Design review of the part built by this model. Coordinates are the model's own, in mm. Coordinates: 2 decimals unless noted, no trailing zeros. Loops run counter-clockwise (first coordinate to the right, second up) from the corner with the lowest first, then second, coordinate; pieces in that order, holes last. Notation, with made-up numbers: M -6,6 L 1,6 A20 ccw 1,32 Z; hole C 43,-1 d8. An arc over 180 degrees is marked long. Answer as a JSON object with one key per item and string values. Group by question number.
1. Consider section C-C (y = 5.5). State the section outline as (x, z) points (3 decimals).
2. Insertion check: pin 1 (0.8 mm diameter, centred on x = 93.5, z = 2.5, fed in from -Y); pin 2 (1 mm diameter, centred on y = 23.5, z = 1, fed in from +X); pin 3 (1 mm diameter, centred on x = 139.5, z = 1.5, fed in from +Y); pin 4 (3.5 mm diameter, centred on x = 104.67, y = 62.3, fed in from +Z) (3 decimals). Each pin has a flat end and moves straight along its axis. Give the tip position at first contact, or say it passes through.
3. To check wall thickness, follow probe 1 along Y at (x, z) = (149, 0.4); probe 2 along Y at (x, z) = (93.5, 1.4); probe 3 along X at (y, z) = (22, 2.05). State the ranges of each line that lie inside material, in increasing order.
4. Consider section B-B (x = 129). State the section outline as (y, z) points (3 decimals), then the cut area to 3 significant figures.
from build123d import *

# Parameters (mm, degrees)
SKETCH1_R           = 1.5875
BOSS_EXTRUDE1_DEPTH = 3.175


with BuildPart() as part:
    # Sketch1 → Boss-Extrude1 (new body)
    with BuildSketch(Plane.XY):
        with BuildLine():
            Line((145.943650407, -28.027444193), (145.943650407, -24.852444193))
            Line((145.943650407, -24.852444193), (152.293650407, -24.852444193))
            Line((152.293650407, -24.852444193), (155.468650407, -24.852444193))
            Line((155.468650407, -24.852444193), (155.468650407, -28.027444193))
            Line((155.468650407, -28.027444193), (155.468650407, -40.727444193))
            Line((155.468650407, -40.727444193), (155.468650407, -43.902444193))
            Line((155.468650407, -43.902444193), (145.943650407, -43.902444193))
            Line((145.943650407, -43.902444193), (145.943650407, -40.727444193))
            ThreePointArc((145.943650407, -40.727444193), (87.543306121, -2.160349908), (100.082539295, 66.693034944))
            ThreePointArc((100.082539295, 66.693034944), (109.06069832, 66.887098142), (109.254761518, 57.908939117))
            ThreePointArc((109.254761518, 57.908939117), (99.104850954, 42.438945049), (95.168461153, 24.360055807))
            Line((95.168461153, 24.360055807), (92.628461153, 24.360055807))
            Line((92.628461153, 24.360055807), (92.628461153, 21.185055807))
            Line((92.628461153, 21.185055807), (95.168461153, 21.185055807))
            ThreePointArc((95.168461153, 21.185055807), (95.286372211, 18.967274494), (95.501106091, 16.756766333))
            ThreePointArc((95.501106091, 16.756766333), (103.592613564, -5.281493426), (120.729197754, -21.328140077))
            Line((120.729197754, -21.328140077), (131.710241083, -27.141852582))
            ThreePointArc((131.710241083, -27.141852582), (133.438776966, -27.802732961), (135.275650407, -28.027444193))
            Line((135.275650407, -28.027444193), (145.943650407, -28.027444193))
        make_face()
        with Locations((104.668650407, 62.300987031)):
            Circle(SKETCH1_R, mode=Mode.SUBTRACT)
    extrude(amount=BOSS_EXTRUDE1_DEPTH)


solid = part.part
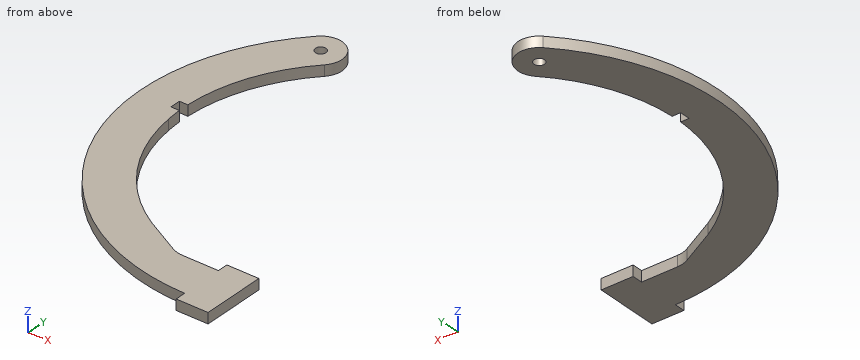
Findings below:
{
 "1": {"outline": "M 84.838,0 L 98.17,0 L 98.17,3.175 L 84.838,3.175 Z"},
 "2": {"pin 1": "stops at y = -13.61", "pin 2": "stops at x = 92.63", "pin 3": "stops at y = -28.03", "pin 4": "stops at z = 3.175"},
 "3": {"probe 1": "y = -43.9 to -24.85", "probe 2": "y = -13.03 to 21.19, 24.36 to 58.58", "probe 3": "x = 82.45 to 92.63"},
 "4": {"outline": "M -38.425,0 L -25.707,0 L -25.707,3.175 L -38.425,3.175 Z", "area": "40.4 mm^2"}
}
